Geometry check sheet. Reference: the model listing, model coordinates, mm. Face numbers are marked on the shaded views. A direction names the side the tool comes from. Coordinates: 2 decimals unless noted, no trailing zeros. Order: outer loops, then holes, each group sorted by start corner. A loop starts at its lowest first (then second) coordinate and runs counter-clockwise, first axis right, second up. Notation, with made-up numbers: (40.5, 76) - (64.5, 76) arc R20 cw to (64.5, 110) - close; hole circle Ø7 at (26.25, 8.5). An arc over 180 degrees is marked (long way). One line per item, written item: value. Start each with the question number.
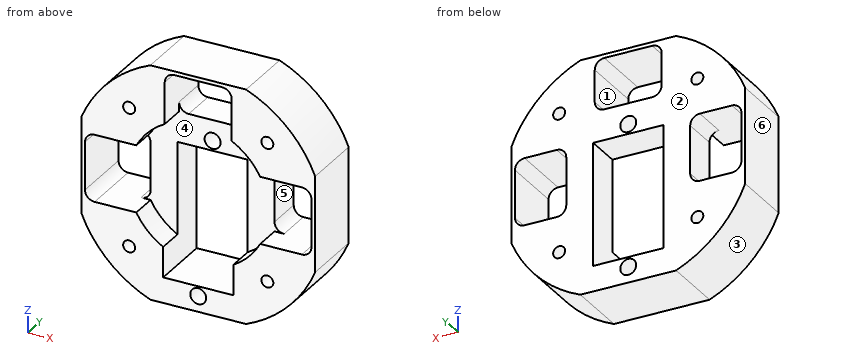
```python
from build123d import *

# Parameters (mm, degrees)
SKETCH2_R           = 1.125
SKETCH2_R_2         = 1.5
SKETCH2_W           = 13.2
SKETCH2_H           = 23.1
BOSS_EXTRUDE3_DEPTH = 11.7
SKETCH2_9_R         = 1.5
CUT_EXTRUDE3_DEPTH  = 5
FILLET1_R           = 1.8


with BuildPart() as part:
    # Sketch2 → Boss-Extrude3 (new body)
    with BuildSketch(Plane(origin=(0, 0, 0), x_dir=(1, 0, 0), z_dir=(0, 1, 0))):
        with BuildLine():
            ThreePointArc((-9, 22), (-16.807736314, 16.807736314), (-22, 9))
            Line((-22, 9), (-22, -9))
            ThreePointArc((-22, -9), (-16.807736314, -16.807736314), (-9, -22))
            Line((-9, -22), (9, -22))
            ThreePointArc((9, -22), (16.807736314, -16.807736314), (22, -9))
            Line((22, -9), (22, 9))
            ThreePointArc((22, 9), (16.807736314, 16.807736314), (9, 22))
            Line((9, 22), (-9, 22))
        make_face()
        with Locations(Location((-13, -13, 0), (0, 0, 270))):
            Circle(SKETCH2_R, mode=Mode.SUBTRACT)
        with BuildLine():
            Line((6.3, -11.65643599), (6.3, -19.5))
            ThreePointArc((6.3, -19.5), (5.772792206, -20.772792206), (4.5, -21.3))
            Line((4.5, -21.3), (-4.5, -21.3))
            ThreePointArc((-4.5, -21.3), (-5.772792206, -20.772792206), (-6.3, -19.5))
            Line((-6.3, -19.5), (-6.3, -11.65643599))
            Line((-6.3, -11.65643599), (6.3, -11.65643599))
        make_face(mode=Mode.SUBTRACT)
        with Locations(Location((13, -13, 0), (0, 0, 270))):
            Circle(SKETCH2_R, mode=Mode.SUBTRACT)
        with Locations(Location((0, -7.75, 0), (0, 0, 270))):
            Circle(SKETCH2_R_2, mode=Mode.SUBTRACT)
        with BuildLine():
            Line((-19.5, 6.3), (-11.65643599, 6.3))
            Line((-11.65643599, 6.3), (-11.65643599, -6.3))
            Line((-11.65643599, -6.3), (-19.5, -6.3))
            ThreePointArc((-19.5, -6.3), (-20.772792206, -5.772792206), (-21.3, -4.5))
            Line((-21.3, -4.5), (-21.3, 4.5))
            ThreePointArc((-21.3, 4.5), (-20.772792206, 5.772792206), (-19.5, 6.3))
        make_face(mode=Mode.SUBTRACT)
        with Locations(Location((0, 19.06, 0), (0, 0, 270))):
            Circle(SKETCH2_R_2, mode=Mode.SUBTRACT)
        with Locations((0, 5.655)):
            Rectangle(SKETCH2_W, SKETCH2_H, mode=Mode.SUBTRACT)
        with BuildLine():
            Line((11.65643599, 6.3), (19.5, 6.3))
            ThreePointArc((19.5, 6.3), (20.772792206, 5.772792206), (21.3, 4.5))
            Line((21.3, 4.5), (21.3, -4.5))
            ThreePointArc((21.3, -4.5), (20.772792206, -5.772792206), (19.5, -6.3))
            Line((19.5, -6.3), (11.65643599, -6.3))
            Line((11.65643599, -6.3), (11.65643599, 6.3))
        make_face(mode=Mode.SUBTRACT)
        with Locations(Location((13, 13, 0), (0, 0, 270))):
            Circle(SKETCH2_R, mode=Mode.SUBTRACT)
        with Locations(Location((-13, 13, 0), (0, 0, 270))):
            Circle(SKETCH2_R, mode=Mode.SUBTRACT)
    extrude(amount=BOSS_EXTRUDE3_DEPTH)

    # Sketch2<9> → Cut-Extrude3 (cut)
    with BuildSketch(Plane(origin=(0, 0, 0), x_dir=(1, 0, 0), z_dir=(0, 1, 0))):
        with BuildLine():
            Line((-6.3, -11.65643599), (6.3, -11.65643599))
            ThreePointArc((6.3, -11.65643599), (9.369164851, -9.369164851), (11.65643599, -6.3))
            Line((11.65643599, -6.3), (11.65643599, 6.3))
            ThreePointArc((11.65643599, 6.3), (9.489805129, 9.246950774), (6.6, 11.489234091))
            Line((6.6, 11.489234091), (6.6, -5.895))
            Line((6.6, -5.895), (-6.6, -5.895))
            Line((-6.6, -5.895), (-6.6, 11.489234091))
            ThreePointArc((-6.6, 11.489234091), (-9.489805129, 9.246950774), (-11.65643599, 6.3))
            Line((-11.65643599, 6.3), (-11.65643599, -6.3))
            ThreePointArc((-11.65643599, -6.3), (-9.369164851, -9.369164851), (-6.3, -11.65643599))
        make_face()
        with Locations(Location((0, -7.75, 0), (0, 0, 270))):
            Circle(SKETCH2_9_R, mode=Mode.SUBTRACT)
    extrude(amount=CUT_EXTRUDE3_DEPTH, mode=Mode.SUBTRACT)

    # Fillet1
    fillet1_edges = [part.edges().sort_by_distance(p)[0] for p in [
        (-11.65643599, 8.35, 6.3),
        (-11.65643599, 8.35, -6.3),
        (6.3, 8.35, 11.65643599),
        (-6.3, 8.35, 11.65643599),
        (11.65643599, 8.35, -6.3),
        (11.65643599, 8.35, 6.3),
    ]]
    fillet(fillet1_edges, radius=FILLET1_R)


solid = part.part
```
Q1. Cross-section at B-B, the plane z = -19.06. Enter the section's corners in (x, y), and give its area (3 significant figures).
Q2. Release check for a two-part mould opening along X. For the marked faces 1, 2 and 3 record: released by +X, released by -X, zero draft, split by the parting line, or undercut.
Q3. Set-up check for the marked faces 4, 5 and 6: record each of +Z, -Z, +X, -X, +Y, -Y from which the full face is reachable in a straight line by a thin tool's end or side.
Q4. Material ranges on probe 1 along X at (y, z) = (8, -1.5); probe 2 along Z at (x, y) = (4.5, 11) (3 decimals); probe 3 along X at (y, z) = (8.75, 7.75), recorded low to high.
Q5. Cross-section at C-C, the plane z = -13. Enter the section's corners in (x, y) (3 decimals).
Q6. Cross-section at A-A, the plane x = 0. Enter the section's corners in (y, z) (3 decimals).
Q7. Gauge pin test, flat ends, axial feed: P1, Ø2, axis at x = 13, z = 13, coming from the -Y side; P2, Ø3, axis at y = 7.5, z = -16.5, coming from the -X side; P3, Ø6, axis at x = 16.5, y = 9.5, coming from the +Z side; P4, Ø5, axis at x = -14.5, y = 1.5, coming from the -Z side. Record the tip position at first contact, or that the pin passes through.
Q8. Cross-section at D-D, the plane y = 1.25. Count the separate pieces of the cut face and the enclosed holes in it, and give its area (3 significant figures).
Check result:
1. outline: (-14.2, 0) - (-1.5, 0) - (-1.5, 11.7) - (-14.2, 11.7) - close; (1.5, 0) - (14.2, 0) - (14.2, 11.7) - (1.5, 11.7) - close
1. area: 297 mm2
2. face 1: undercut
2. face 2: zero draft
2. face 3: released by -X
3. face 4: -Y
3. face 5: +Y, -Y
3. face 6: +Z, -Z, -X, +Y, -Y
4. probe 1: x = -22 to -21.3, -11.66 to -6.6, 6.6 to 11.66, 21.3 to 22
4. probe 2: z = -22 to -17.205, 5.895 to 11.656, 21.3 to 22
4. probe 3: x = -22 to -1.5, 1.5 to 22
5. outline: (-19.9, 0) - (-14.125, 0) - (-14.125, 11.7) - (-19.9, 11.7) - close; (-11.875, 0) - (-6.6, 0) - (-6.6, 11.7) - (-11.875, 11.7) - close; (6.6, 0) - (11.875, 0) - (11.875, 11.7) - (6.6, 11.7) - close; (14.125, 0) - (19.9, 0) - (19.9, 11.7) - (14.125, 11.7) - close
6. outline: (0, -22) - (11.7, -22) - (11.7, -20.56) - (0, -20.56) - close; (0, -17.56) - (11.7, -17.56) - (11.7, -17.205) - (0, -17.205) - close; (0, 21.3) - (11.7, 21.3) - (11.7, 22) - (0, 22) - close; (5, 5.895) - (11.7, 5.895) - (11.7, 6.25) - (5, 6.25) - close; (5, 9.25) - (11.7, 9.25) - (11.7, 11.656) - (5, 11.656) - close
7. P1: passes through
7. P2: stops at x = -18.44
7. P3: stops at z = 19.56
7. P4: stops at z = -20.52
8. separate pieces: 1
8. enclosed holes: 6
8. area: 735 mm2
